Input: part model. Units: mm. Frame: model coordinates. A direction names the side the tool comes from. Coordinates: 2 decimals unless noted, no trailing zeros. Write each loop counter-clockwise with the first axis right and the second up, starting at its lowest first coordinate (ties: lowest second). Pieces come first, ordered by that corner, then holes.
1) Set-up query: faces 1 (the flat face through (33, 3, -25)), 2 (the cylindrical face through (38.266, 24.269, 1.021)), 3 (the cylindrical face through (30.89, 2.54, -37.36)), 4 (the flat face through (16, 5, -27)), 5 (the flat face through (7, 22, 2.5)). Return all of +Z, -Z, +X, -X, +Y, -Y with unobstructed straight access to the full face (end or side cutting, diameter ignored); none if empty.
2) Line query: L1, parallel to X at y = 4, z = -3.75; L2, parallel to X at y = 13.65, z = -3.75; L3, parallel to X at y = 19.25, z = 0. Output: solid intervals per line, ascending.
3) Section query C-C (x = 11.5). Output: boundary loops of the cut face in (y, z).
4) Pin query (flat end, axial travel): pin 1 Ø2.5 at (x, y) = (8.64, 21) entering from +Z; pin 2 Ø1.5 at (x, z) = (30, -8) entering from +Y; pin 3 Ø15.5 at (x, z) = (19.5, -20) entering from +Y; pin 4 Ø2 at (x, z) = (29.5, -38.25) entering from -Y. Return the tip coordinate at first contact, or that it passes through.
5) Section query B-B (y = 17.75). Output: boundary loops of the cut face in (x, z).
6) Section query A-A (z = 0.5). Output: boundary loops of the cut face in (x, y).
7) Draft query along X for faces 6 (the flat face through (10.7, 20, 1)), 7 (the cylindrical face through (38.4, 7.4, -6.92)), 8 (the flat face through (28, 12, -2)), 9 (the flat face through (0, 4, -12)). Return one class per face: pulls with the +X half, pulls with the -X half, needs draft (parallel to the pull), parting line crosses it, or undercut.
8) Section query D-D (y = 13.5). Output: boundary loops of the cut face in (x, z).
from build123d import *

# Parameters (mm, degrees)
SKETCH1_W           = 33
SKETCH1_H           = 42
BOSS_EXTRUDE1_DEPTH = 5
SKETCH4_R           = 1.65
CUT_EXTRUDE1_DEPTH  = 10
SKETCH6_W           = 6
SKETCH6_H           = 7.490694283
BOSS_EXTRUDE2_DEPTH = 5
BOSS_EXTRUDE4_START = 10
SKETCH8_R           = 1.65
BOSS_EXTRUDE4_DEPTH = 10
SKETCH9_W           = 4.9
SKETCH9_H           = 3
BOSS_EXTRUDE5_DEPTH = 10
FILLET2_R           = 2.5
CUT_EXTRUDE3_DEPTH  = 10
SKETCH11_W          = 33
SKETCH11_H          = 34.509305717
CUT_EXTRUDE4_DEPTH  = 10
FILLET3_R           = 4
FILLET4_R           = 2
FILLET5_R           = 4
SKETCH12_R          = 3.5
CUT_EXTRUDE5_DEPTH  = 3
SKETCH13_W          = 4.5
SKETCH13_H          = 3
BOSS_EXTRUDE6_DEPTH = 12
FILLET6_R           = 2
CUT_EXTRUDE6_DEPTH  = 7
CHAMFER1_SIZE       = 2


# Some blends are built 0.0001 mm under size
with BuildPart() as part:
    # Sketch1 → Boss-Extrude1 (new body)
    with BuildSketch(Plane(origin=(0, 0, 0), x_dir=(1, 0, 0), z_dir=(0, 1, 0))):
        with Locations((16.5, 21)):
            Rectangle(SKETCH1_W, SKETCH1_H)
    extrude(amount=BOSS_EXTRUDE1_DEPTH)

    # Sketch4 → Cut-Extrude1 (cut)
    with BuildSketch(Plane(origin=(0, 5, 0), x_dir=(1, 0, 0), z_dir=(0, 1, 0))):
        with Locations(Location((4.500000179, 3.75, 0), (0, 0, 270))):
            Circle(SKETCH4_R)
        with Locations(Location((3.500000179, 38.249999434, 0), (0, 0, 270))):
            Circle(SKETCH4_R)
        with Locations(Location((29.5, 38.249999434, 0), (0, 0, 270))):
            Circle(SKETCH4_R)
        with Locations(Location((28.5, 3.75, 0), (0, 0, 270))):
            Circle(SKETCH4_R)
    extrude(amount=-CUT_EXTRUDE1_DEPTH, mode=Mode.SUBTRACT)

    # Sketch6 → Boss-Extrude2 (add)
    with BuildSketch(Plane(origin=(0, 5, 0), x_dir=(1, 0, 0), z_dir=(0, 1, 0))):
        with Locations((36, 3.745347142)):
            Rectangle(SKETCH6_W, SKETCH6_H)
        Polygon((0, -5), (0, 0), (33, 0), (39, 0), (39, -5), align=None)
    extrude(amount=-BOSS_EXTRUDE2_DEPTH)

    # Sketch8 → Boss-Extrude4 (add)
    with BuildSketch(Plane(origin=(0, 5, 0), x_dir=(1, 0, 0), z_dir=(0, 1, 0)).offset(BOSS_EXTRUDE4_START)):
        Polygon((39, 7.490694283), (33, 7.490694283), (33, 42), (0, 42), (0, -5), (39, -5), align=None)
        with Locations(Location((29.5, 38.249999434, 0), (0, 0, 270))):
            Circle(SKETCH8_R, mode=Mode.SUBTRACT)
        with Locations(Location((3.500000179, 38.249999434, 0), (0, 0, 270))):
            Circle(SKETCH8_R, mode=Mode.SUBTRACT)
        with Locations(Location((4.500000179, 3.75, 0), (0, 0, 270))):
            Circle(SKETCH8_R, mode=Mode.SUBTRACT)
        with Locations(Location((28.5, 3.75, 0), (0, 0, 270))):
            Circle(SKETCH8_R, mode=Mode.SUBTRACT)
    extrude(amount=-BOSS_EXTRUDE4_DEPTH)

    # Sketch9 → Boss-Extrude5 (add)
    with BuildSketch(Plane(origin=(0, 15, 0), x_dir=(1, 0, 0), z_dir=(0, 1, 0))):
        with Locations((36.55, -1)):
            Rectangle(SKETCH9_W, SKETCH9_H)
    extrude(amount=BOSS_EXTRUDE5_DEPTH)

    # Fillet2
    # the kernel refuses this fillet: 2.5 mm, written as the material it takes off along each edge
    with BuildSketch(Plane(origin=(34.1, 25, -6.75), x_dir=(0, -1, 0), z_dir=(0, 0, 1)), Plane(origin=(39, 25, 8.75), x_dir=(0, -1, 0), z_dir=(0, 0, -1))) as fillet2_piece_1:
        with BuildLine():
            CenterArc((FILLET2_R, FILLET2_R), FILLET2_R, 180, 90)
            Line((0, FILLET2_R), (0, 0))
            Line((0, 0), (FILLET2_R, 0))
        make_face()
    extrude(amount=15.5, mode=Mode.SUBTRACT)

    # Sketch10 → Cut-Extrude3 (cut)
    with BuildSketch(Plane(origin=(0, 0, -0.5), x_dir=(-1, 0, 0), z_dir=(0, 0, -1))):
        with BuildLine():
            ThreePointArc((-37.068227721, 21.5), (-37.194918455, 21), (-37.068227721, 20.5))
            ThreePointArc((-37.068227721, 20.5), (-35.887018018, 19.982165355), (-35.094918455, 21))
            ThreePointArc((-35.094918455, 21), (-35.887018018, 22.017834645), (-37.068227721, 21.5))
        make_face()
    extrude(amount=-CUT_EXTRUDE3_DEPTH, mode=Mode.SUBTRACT)

    # Sketch11 → Cut-Extrude4 (cut)
    with BuildSketch(Plane(origin=(0, 15, 0), x_dir=(1, 0, 0), z_dir=(0, 1, 0))):
        with Locations((16.5, 24.745347142)):
            Rectangle(SKETCH11_W, SKETCH11_H)
    extrude(amount=-CUT_EXTRUDE4_DEPTH, mode=Mode.SUBTRACT)

    # Fillet3
    fillet3_edges = [part.edges().sort_by_distance(p)[0] for p in [
        (0, 2.5, -42),
        (33, 2.5, -42),
        (33, 2.5, -7.490694283),
    ]]
    fillet(fillet3_edges, radius=FILLET3_R)

    # Fillet4
    fillet4_edges = [part.edges().sort_by_distance(p)[0] for p in [
        (39, 7.5, -7.490694283),
    ]]
    fillet(fillet4_edges, radius=FILLET4_R - 0.0001)  # a hair under: the kernel refuses the full size

    # Fillet5
    fillet5_edges = [part.edges().sort_by_distance(p)[0] for p in [
        (18.5, 5, -7.490694283),
    ]]
    fillet(fillet5_edges, radius=FILLET5_R)

    # Sketch12 → Cut-Extrude5 (cut)
    with BuildSketch(Plane(origin=(0, 15, 0), x_dir=(1, 0, 0), z_dir=(0, 1, 0))):
        with Locations(Location((4.500000179, 3.75, 0), (0, 0, 270))):
            Circle(SKETCH12_R)
        with Locations(Location((28.5, 3.75, 0), (0, 0, 270))):
            Circle(SKETCH12_R)
    extrude(amount=-CUT_EXTRUDE5_DEPTH, mode=Mode.SUBTRACT)

    # Sketch13 → Boss-Extrude6 (add)
    with BuildSketch(Plane(origin=(0, 15, 0), x_dir=(1, 0, 0), z_dir=(0, 1, 0))):
        with Locations((8.45, -1)):
            Rectangle(SKETCH13_W, SKETCH13_H)
    extrude(amount=BOSS_EXTRUDE6_DEPTH)

    # Fillet6
    fillet6_edges = [part.edges().sort_by_distance(p)[0] for p in [
        (6.2, 27, 1),
        (10.7, 27, 1),
    ]]
    fillet(fillet6_edges, radius=FILLET6_R)

    # Sketch14 → Cut-Extrude6 (cut)
    with BuildSketch(Plane(origin=(0, 0, -0.5), x_dir=(-1, 0, 0), z_dir=(0, 0, -1))):
        with BuildLine():
            ThreePointArc((-7.594918455, 21), (-7.62708381, 21.257900437), (-7.721609189, 21.5))
            ThreePointArc((-7.721609189, 21.5), (-9.694918455, 21), (-7.721609189, 20.5))
            ThreePointArc((-7.721609189, 20.5), (-7.62708381, 20.742099563), (-7.594918455, 21))
        make_face()
    extrude(amount=-CUT_EXTRUDE6_DEPTH, mode=Mode.SUBTRACT)

    # Chamfer1
    chamfer1_edges = [part.edges().sort_by_distance(p)[0] for p in [
        (8.45, 15, 2.5),
        (36.55, 15, 2.5),
    ]]
    chamfer(chamfer1_edges, length=CHAMFER1_SIZE)


solid = part.part
Answer:
1. face 1: -Z, +X, +Y, -Y
1. face 2: +Z, -Z, +X, +Y
1. face 3: +Y, -Y
1. face 4: -Z, +X, -X, +Y
1. face 5: +Z, +X, -X, +Y
2. L1: x = 0 to 2.85, 6.15 to 26.85, 30.15 to 39
2. L2: x = 0 to 1, 8 to 25, 32 to 39
2. L3: x = 6.2 to 10.7, 34.1 to 39
3. outline: (0, -42) - (5, -42) - (5, -11.49) arc R4 cw to (9, -7.49) - (15, -7.49) - (15, 5) - (0, 5) - close
4. pin 1: stops at z = 2.5
4. pin 2: stops at y = 15
4. pin 3: stops at y = 5
4. pin 4: passes through
5. outline: (6.2, -0.5) - (10.7, -0.5) - (10.7, 2.5) - (6.2, 2.5) - close; (34.1, -0.5) - (39, -0.5) - (39, 2.5) - (34.1, 2.5) - close
6. outline: (0, 0) - (39, 0) - (39, 22.5) arc R2.5 ccw to (36.55, 25) arc R2.5 ccw to (34.1, 22.5) - (34.1, 15) - (10.7, 15) - (10.7, 25) arc R2 ccw to (8.7, 27) - (8.2, 27) arc R2 ccw to (6.2, 25) - (6.2, 15) - (0, 15) - close; hole circle Ø2.1 at (8.64, 21); hole circle Ø2.1 at (36.14, 21)
7. face 6: undercut
7. face 7: pulls with the +X half
7. face 8: undercut
7. face 9: pulls with the -X half
8. outline: (0, -7.49) - (37, -7.49) arc R2 ccw to (39, -5.49) - (39, 5) - (0, 5) - close; hole circle Ø7 at (4.5, -3.75); hole circle Ø7 at (28.5, -3.75)
